```python
from build123d import *

# Parameters (mm, degrees)
SKETCH_1_R      = 13.5
SKETCH_1_R_2    = 2.15
SKETCH_1_R_3    = 1.3
EXTRUDE_1_DEPTH = 5
FILLET_1_R      = 2


with BuildPart() as part:
    # ｽｹｯﾁ1 → ﾎﾞｽ - 押し出し1 (new body)
    with BuildSketch(Plane(origin=(0, 0, 0), x_dir=(1, 0, 0), z_dir=(0, 1, 0))):
        with BuildLine():
            Line((-24.445436483, -32.25), (-24.445436483, -19.445436483))
            ThreePointArc((-24.445436483, -19.445436483), (-23.793249982, -16.976323733), (-22.006829374, -15.151339784))
            ThreePointArc((-22.006829374, -15.151339784), (-19.398069264, -11.924552334), (-19.507056212, -7.776551803))
            ThreePointArc((-19.507056212, -7.776551803), (-21, 0), (-19.507056212, 7.776551803))
            ThreePointArc((-19.507056212, 7.776551803), (-19.398069264, 11.924552334), (-22.006829374, 15.151339784))
            ThreePointArc((-22.006829374, 15.151339784), (-22.980970389, 22.980970389), (-15.151339784, 22.006829374))
            ThreePointArc((-15.151339784, 22.006829374), (-11.924552334, 19.398069264), (-7.776551803, 19.507056212))
            ThreePointArc((-7.776551803, 19.507056212), (0, 21), (7.776551803, 19.507056212))
            ThreePointArc((7.776551803, 19.507056212), (11.924552334, 19.398069264), (15.151339784, 22.006829374))
            ThreePointArc((15.151339784, 22.006829374), (22.980970389, 22.980970389), (22.006829374, 15.151339784))
            ThreePointArc((22.006829374, 15.151339784), (19.398069264, 11.924552334), (19.507056212, 7.776551803))
            ThreePointArc((19.507056212, 7.776551803), (21, 0), (19.507056212, -7.776551803))
            ThreePointArc((19.507056212, -7.776551803), (19.398069264, -11.924552334), (22.006829374, -15.151339784))
            ThreePointArc((22.006829374, -15.151339784), (23.793249982, -16.976323733), (24.445436483, -19.445436483))
            Line((24.445436483, -19.445436483), (24.445436483, -32.25))
            Line((24.445436483, -32.25), (14.953214466, -32.25))
            Line((14.953214466, -32.25), (14.953214466, -37.25))
            Line((14.953214466, -37.25), (-19.445436483, -37.25))
            ThreePointArc((-19.445436483, -37.25), (-22.980970389, -35.785533906), (-24.445436483, -32.25))
        make_face()
        with Locations(Location((0, 0, 0), (0, 0, 270))):
            Circle(SKETCH_1_R, mode=Mode.SUBTRACT)
        with Locations(Location((12.374368671, 12.374368671, 0), (0, 0, 270))):
            Circle(SKETCH_1_R_2, mode=Mode.SUBTRACT)
        with Locations(Location((12.374368671, -12.374368671, 0), (0, 0, 270))):
            Circle(SKETCH_1_R_2, mode=Mode.SUBTRACT)
        with Locations(Location((-12.374368671, -12.374368671, 0), (0, 0, 270))):
            Circle(SKETCH_1_R_2, mode=Mode.SUBTRACT)
        with Locations(Location((-12.374368671, 12.374368671, 0), (0, 0, 270))):
            Circle(SKETCH_1_R_2, mode=Mode.SUBTRACT)
        with Locations(Location((19.445436483, 19.445436483, 0), (0, 0, 270))):
            Circle(SKETCH_1_R_2, mode=Mode.SUBTRACT)
        with Locations(Location((19.445436483, -19.445436483, 0), (0, 0, 270))):
            Circle(SKETCH_1_R_2, mode=Mode.SUBTRACT)
        with Locations(Location((-19.445436483, -19.445436483, 0), (0, 0, 270))):
            Circle(SKETCH_1_R_2, mode=Mode.SUBTRACT)
        with Locations(Location((-19.445436483, 19.445436483, 0), (0, 0, 270))):
            Circle(SKETCH_1_R_2, mode=Mode.SUBTRACT)
        with Locations(Location((7.554563517, -31, 0), (0, 0, 270))):
            Circle(SKETCH_1_R_3, mode=Mode.SUBTRACT)
        with Locations(Location((-18.445436483, -31, 0), (0, 0, 270))):
            Circle(SKETCH_1_R_3, mode=Mode.SUBTRACT)
    extrude(amount=EXTRUDE_1_DEPTH)

    # ﾌｨﾚｯﾄ1
    fillet_1_edges = [part.edges().sort_by_distance(p)[0] for p in [
        (24.445436483, 2.5, 32.25),
        (14.953214466, 2.5, 32.25),
        (14.953214466, 2.5, 37.25),
    ]]
    fillet(fillet_1_edges, radius=FILLET_1_R)


solid = part.part
```
Check sheet for the modelled part. Datum: model origin and axes. Units: mm. A direction names the side the tool comes from. Give positions to 0.01 mm unless a question says otherwise; leave off trailing zeros. Loops run counter-clockwise (first coordinate to the right, second up) from the corner with the lowest first, then second, coordinate; pieces in that order, holes last. Notation, with made-up numbers: (61.5, 10) - (100.5, 10) arc R15 ccw to (100.5, 26) - close; hole circle Ø9 at (85.25, -26.5). An arc over 180 degrees is marked (long way). One line per question, with ' | ' between items. Start each with the question number.
1. Cross-section at C-C, the plane z = 31. Enter the section's corners in (x, y), plus the area to 3 significant figures.
2. Draft check along X on faces 3 (the cylindrical face through (-19.38, 2.46, -11.87)), 4 (the cylindrical face through (11.87, 2.46, -19.38)), 5 (the cylindrical face through (23.844, 2.535, 31.68)). Enter one of: released by +X, released by -X, zero draft, split by the parting line, or undercut.
3. Set-up check for faces 1 (the flat face through (-24.445, 2, 26)), 2 (the flat face through (20, 2, 32.25)): record each of +Z, -Z, +X, -X, +Y, -Y from which the full face is reachable in a straight line by a thin tool's end or side.
4. Cross-section at B-B, the plane x = 0. Enter the section's corners in (y, z).
5. Material ranges on line 1 along X through (y, z) = (3.75, -14); line 2 along X through (y, z) = (3.5, 21); line 3 along X through (y, z) = (3.85, 1), recorded low to high. Write a range as [from, to].
6. Cross-section at A-A, the plane z = 0. Enter the section's corners in (x, y), plus the area to 3 significant figures.
7. Gauge pin test, flat ends, axial feed: pin 1 Ø4 at (x, z) = (19.45, -19.45) entering from +Y; pin 2 Ø2 at (y, z) = (3, 6.5) entering from +X; pin 3 Ø0.8 at (y, z) = (3.5, 35) entering from +X. Record the tip position at first contact, or that the pin passes through.
8. Cross-section at D-D, the plane y = 2. Give the number of separate pieces and of enclosed holes in the cut face, plus the area to 3 significant figures.
Check result:
1) outline: (-24.45, 0) - (-19.75, 0) - (-19.75, 5) - (-24.45, 5) - close; (-17.15, 0) - (6.25, 0) - (6.25, 5) - (-17.15, 5) - close; (8.85, 0) - (24.3, 0) - (24.3, 5) - (8.85, 5) - close | area: 218 mm2
2) face 3: released by -X | face 4: undercut | face 5: released by +X
3) face 1: +Z, -Z, -X, +Y, -Y | face 2: +Z, +X, +Y, -Y
4) outline: (0, -21) - (5, -21) - (5, -13.5) - (0, -13.5) - close; (0, 13.5) - (5, 13.5) - (5, 37.25) - (0, 37.25) - close
5) line 1: x = [-20.61, -13.78], [-10.97, 10.97], [13.78, 20.61] | line 2: x = [-24.45, -20.93], [-17.96, 17.96], [20.93, 24.45] | line 3: x = [-20.98, -13.46], [13.46, 20.98]
6) outline: (-21, 0) - (-13.5, 0) - (-13.5, 5) - (-21, 5) - close; (13.5, 0) - (21, 0) - (21, 5) - (13.5, 5) - close | area: 75.0 mm2
7) pin 1: passes through | pin 2: stops at x = 20.27 | pin 3: stops at x = 14.95
8) separate pieces: 1 | enclosed holes: 11 | area: 1,840 mm2
